For this review, take the finished solid that the model builds, in its own axes (mm). A direction names the side the tool comes from. Coordinates: 2 decimals unless noted, no trailing zeros. Order: outer loops, then holes, each group sorted by start corner. A loop starts at its lowest first (then second) coordinate and runs counter-clockwise, first axis right, second up. Notation, with made-up numbers: (50.25, 25.5) -> (103.25, 25.5) arc R5 cw to (103.25, 32.5) -> close; hole circle Ø5 at (78.5, 8.25). An arc over 180 degrees is marked (long way). Answer as a JSON object with one key per item and string values. Group by question number.
1) Machinability: for faces 1 (the flat face through (-32, -16, 59)), 2 (the flat face through (-37.5, -17, 64)), 3 (the flat face through (-40, -17, 64)), which of the approach directions +Z, -Z, +X, -X, +Y, -Y give a long, thin tool a straight path to every point of the face, cutting with its end or side? Answer none if there is none.
2) Add section A-A, the plane y = -16. Write out the cut boundary in (x, z).
3) Add section C-C, the plane z = 61.25. Write out the cut boundary in (x, y).
4) Add section D-D, the plane z = 62.25. Write out the cut boundary in (x, y), then the cut area to 3 significant figures.
5) Draft analysis for pull direction Z (two halves, no side actions). For faces 4 (the flat face through (-44, -16, 59)), 5 (the flat face through (-39, -16, 55.9)), 6 (the cylindrical face through (-37.92, -16.46, 59.29)), 7 (the cylindrical face through (-34.712, -17.341, 57.167)), state which applies: +Z half, -Z half, draft (parallel to the pull), parting line (faces both ways), or undercut.
6) Add section B-B, the plane x = -39.25. Write out the cut boundary in (y, z), then the cut area to 3 significant figures.
7) For pin 1 (4 mm diameter, centred on x = -42.5, z = 63.5, fed in from +Y); pin 2 (6 mm diameter, centred on x = -35, y = -18.5, fed in from -Z); pin 3 (2 mm diameter, centred on x = -37.5, y = -12, fed in from -Z); pin 4 (1 mm diameter, centred on x = -42, y = -17.5, fed in from +Z), all flat-tipped, find the tip position at first contact; note any pin that passes through.
8) Wall thickness on L1, parallel to Y at x = -41.5, z = 60.4; L2, parallel to X at y = -19.25, z = 62.5; L3, parallel to Y at x = -41, z = 60.75: over which ranges is each line inside the solid? List them lowest first.
from build123d import *

# Parameters (mm, degrees)
SK_BARRIL_R        = 3.5
SK_BARRIL_R_2      = 1.2
BARRIL_DEPTH       = 12
CONTRATUERCA_START = 2.5
SK_CONTRATUERCA_R  = 1.2
CONTRATUERCA_DEPTH = 2.5


with BuildPart() as part:
    # Sk_barril → Barril (new body)
    with BuildSketch(Plane(origin=(-32, 0, 0), x_dir=(0, 0, -1), z_dir=(1, 0, 0))):
        with Locations((-60.4, -16)):
            Circle(SK_BARRIL_R)
        with Locations((-60.4, -16)):
            Circle(SK_BARRIL_R_2, mode=Mode.SUBTRACT)
    extrude(amount=-BARRIL_DEPTH)

    # Sk_contratuerca → Contratuerca (add)
    with BuildSketch(Plane(origin=(-40, 0, 0), x_dir=(0, 0, -1), z_dir=(1, 0, 0)).offset(CONTRATUERCA_START)):
        Polygon((-60.4, -10.803847577), (-64.9, -13.401923789), (-64.9, -18.598076211), (-60.4, -21.196152423), (-55.9, -18.598076211), (-55.9, -13.401923789), align=None)
        with Locations((-60.4, -16)):
            Circle(SK_CONTRATUERCA_R, mode=Mode.SUBTRACT)
    extrude(amount=-CONTRATUERCA_DEPTH)


solid = part.part
Output values:
{
 "1": {"face 1": "+Z, -Z, +X, +Y, -Y", "face 2": "+X", "face 3": "-X"},
 "2": {"outline": "(-44, 56.9) -> (-40, 56.9) -> (-40, 55.9) -> (-37.5, 55.9) -> (-37.5, 56.9) -> (-32, 56.9) -> (-32, 59.2) -> (-44, 59.2) -> close; (-44, 61.6) -> (-32, 61.6) -> (-32, 63.9) -> (-37.5, 63.9) -> (-37.5, 64.9) -> (-40, 64.9) -> (-40, 63.9) -> (-44, 63.9) -> close"},
 "3": {"outline": "(-44, -19.4) -> (-40, -19.4) -> (-40, -20.71) -> (-37.5, -20.71) -> (-37.5, -19.4) -> (-32, -19.4) -> (-32, -16.85) -> (-44, -16.85) -> close; (-44, -15.15) -> (-32, -15.15) -> (-32, -12.6) -> (-37.5, -12.6) -> (-37.5, -11.29) -> (-40, -11.29) -> (-40, -12.6) -> (-44, -12.6) -> close"},
 "4": {"outline": "(-44, -18.97) -> (-40, -18.97) -> (-40, -20.13) -> (-37.5, -20.13) -> (-37.5, -18.97) -> (-32, -18.97) -> (-32, -13.03) -> (-37.5, -13.03) -> (-37.5, -11.87) -> (-40, -11.87) -> (-40, -13.03) -> (-44, -13.03) -> close", "area": "77.1 mm²"},
 "5": {"face 4": "draft", "face 5": "-Z half", "face 6": "undercut", "face 7": "parting line"},
 "6": {"outline": "(-21.2, 60.4) -> (-18.6, 55.9) -> (-13.4, 55.9) -> (-10.8, 60.4) -> (-13.4, 64.9) -> (-18.6, 64.9) -> close; hole circle Ø2.4 at (-16, 60.4)", "area": "65.6 mm²"},
 "7": {"pin 1": "stops at y = -12.68", "pin 2": "stops at z = 55.9", "pin 3": "stops at z = 56.6", "pin 4": "stops at z = 63.75"},
 "8": {"L1": "y = -19.5 to -17.2, -14.8 to -12.5", "L2": "x = -40 to -37.5", "L3": "y = -19.48 to -17.15, -14.85 to -12.52"}
}
